For this review, take the finished solid that the model builds, in its own axes (mm). A direction names the side the tool comes from. Round coordinates to 2 decimals unless told otherwise and drop trailing zeros. Put each result on its own line as item: value.
from build123d import *

# Parameters (mm, degrees)
SKETCH_1_W          = 140
SKETCH_1_H          = 20.2
SKETCH_1_R          = 3
SKETCH_1_R_2        = 2.5
EXTRUDE_1_DEPTH     = 5
CUT_EXTRUDE_1_DEPTH = 41


with BuildPart() as part:
    # 스케치1 → 돌출1 (new body)
    with BuildSketch(Plane.XY):
        with Locations((12.953994506, 0)):
            Rectangle(SKETCH_1_W, SKETCH_1_H)
        with Locations((-47.044353904, 0)):
            Circle(SKETCH_1_R, mode=Mode.SUBTRACT)
        with Locations((12.955646096, 0)):
            Circle(SKETCH_1_R, mode=Mode.SUBTRACT)
        with Locations((42.953994506, 0)):
            Circle(SKETCH_1_R_2, mode=Mode.SUBTRACT)
        with Locations((72.953994506, 0)):
            Circle(SKETCH_1_R, mode=Mode.SUBTRACT)
        with BuildLine():
            Line((-16.044353904, 5), (-18.044353904, 5))
            ThreePointArc((-18.044353904, 5), (-23.044353904, 0), (-18.044353904, -5))
            Line((-18.044353904, -5), (-16.044353904, -5))
            ThreePointArc((-16.044353904, -5), (-11.044353904, 0), (-16.044353904, 5))
        make_face(mode=Mode.SUBTRACT)
        with BuildLine():
            Line((-16.044353904, 7.5), (-18.044353904, 7.5))
            ThreePointArc((-18.044353904, 7.5), (-19.044353904, 8.5), (-18.044353904, 9.5))
            Line((-18.044353904, 9.5), (-16.044353904, 9.5))
            ThreePointArc((-16.044353904, 9.5), (-15.044353904, 8.5), (-16.044353904, 7.5))
        make_face(mode=Mode.SUBTRACT)
        with BuildLine():
            Line((-10.683137972, -5.25), (-8.683137972, -5.25))
            ThreePointArc((-8.683137972, -5.25), (-7.683137972, -4.25), (-8.683137972, -3.25))
            Line((-8.683137972, -3.25), (-10.683137972, -3.25))
            ThreePointArc((-10.683137972, -3.25), (-11.683137972, -4.25), (-10.683137972, -5.25))
        make_face(mode=Mode.SUBTRACT)
        with BuildLine():
            Line((-9.620718033, -1), (-7.467989775, -1))
            ThreePointArc((-7.467989775, -1), (-6.543625234, 0.036752017), (-7.544353904, 1))
            Line((-7.544353904, 1), (-9.544353904, 1))
            ThreePointArc((-9.544353904, 1), (-10.545082573, 0.036752017), (-9.620718033, -1))
        make_face(mode=Mode.SUBTRACT)
        with BuildLine():
            Line((-20.294353904, 8.361215932), (-22.294353904, 8.361215932))
            ThreePointArc((-22.294353904, 8.361215932), (-23.294353904, 7.361215932), (-22.294353904, 6.361215932))
            Line((-22.294353904, 6.361215932), (-20.294353904, 6.361215932))
            ThreePointArc((-20.294353904, 6.361215932), (-19.294353904, 7.361215932), (-20.294353904, 8.361215932))
        make_face(mode=Mode.SUBTRACT)
        with BuildLine():
            Line((-23.405569836, 5.25), (-25.405569836, 5.25))
            ThreePointArc((-25.405569836, 5.25), (-26.405569836, 4.25), (-25.405569836, 3.25))
            Line((-25.405569836, 3.25), (-23.405569836, 3.25))
            ThreePointArc((-23.405569836, 3.25), (-22.405569836, 4.25), (-23.405569836, 5.25))
        make_face(mode=Mode.SUBTRACT)
        with BuildLine():
            Line((-24.544353904, 1), (-26.544353904, 1))
            ThreePointArc((-26.544353904, 1), (-27.545082573, 0.036752017), (-26.620718033, -1))
            Line((-26.620718033, -1), (-24.467989775, -1))
            ThreePointArc((-24.467989775, -1), (-23.543625234, 0.036752017), (-24.544353904, 1))
        make_face(mode=Mode.SUBTRACT)
        with BuildLine():
            Line((-10.683137972, 3.25), (-8.683137972, 3.25))
            ThreePointArc((-8.683137972, 3.25), (-7.683137972, 4.25), (-8.683137972, 5.25))
            Line((-8.683137972, 5.25), (-10.683137972, 5.25))
            ThreePointArc((-10.683137972, 5.25), (-11.683137972, 4.25), (-10.683137972, 3.25))
        make_face(mode=Mode.SUBTRACT)
        with BuildLine():
            Line((-13.794353904, 6.361215932), (-11.794353904, 6.361215932))
            ThreePointArc((-11.794353904, 6.361215932), (-10.794353904, 7.361215932), (-11.794353904, 8.361215932))
            Line((-11.794353904, 8.361215932), (-13.794353904, 8.361215932))
            ThreePointArc((-13.794353904, 8.361215932), (-14.794353904, 7.361215932), (-13.794353904, 6.361215932))
        make_face(mode=Mode.SUBTRACT)
        with BuildLine():
            Line((-23.405569836, -3.25), (-25.405569836, -3.25))
            ThreePointArc((-25.405569836, -3.25), (-26.405569836, -4.25), (-25.405569836, -5.25))
            Line((-25.405569836, -5.25), (-23.405569836, -5.25))
            ThreePointArc((-23.405569836, -5.25), (-22.405569836, -4.25), (-23.405569836, -3.25))
        make_face(mode=Mode.SUBTRACT)
        with BuildLine():
            Line((-13.794353904, -8.361215932), (-11.794353904, -8.361215932))
            ThreePointArc((-11.794353904, -8.361215932), (-10.794353904, -7.361215932), (-11.794353904, -6.361215932))
            Line((-11.794353904, -6.361215932), (-13.794353904, -6.361215932))
            ThreePointArc((-13.794353904, -6.361215932), (-14.794353904, -7.361215932), (-13.794353904, -8.361215932))
        make_face(mode=Mode.SUBTRACT)
        with BuildLine():
            Line((-20.294353904, -6.361215932), (-22.294353904, -6.361215932))
            ThreePointArc((-22.294353904, -6.361215932), (-23.294353904, -7.361215932), (-22.294353904, -8.361215932))
            Line((-22.294353904, -8.361215932), (-20.294353904, -8.361215932))
            ThreePointArc((-20.294353904, -8.361215932), (-19.294353904, -7.361215932), (-20.294353904, -6.361215932))
        make_face(mode=Mode.SUBTRACT)
        with BuildLine():
            Line((-16.044353904, -9.5), (-18.044353904, -9.5))
            ThreePointArc((-18.044353904, -9.5), (-19.044353904, -8.5), (-18.044353904, -7.5))
            Line((-18.044353904, -7.5), (-16.044353904, -7.5))
            ThreePointArc((-16.044353904, -7.5), (-15.044353904, -8.5), (-16.044353904, -9.5))
        make_face(mode=Mode.SUBTRACT)
    extrude(amount=EXTRUDE_1_DEPTH)

    # 스케치8 → 컷-돌출1 (cut)
    with BuildSketch(Plane.XZ.offset(10.1)):
        with BuildLine():
            ThreePointArc((77.953994506, 2.5), (79.453994506, 1), (80.953994506, 2.5))
            Line((80.953994506, 2.5), (77.953994506, 2.5))
        make_face()
        with BuildLine():
            Line((77.953994506, 2.5), (80.953994506, 2.5))
            ThreePointArc((80.953994506, 2.5), (79.453994506, 4), (77.953994506, 2.5))
        make_face()
        with BuildLine():
            ThreePointArc((61.453994506, 2.5), (62.953994506, 1), (64.453994506, 2.5))
            Line((64.453994506, 2.5), (61.453994506, 2.5))
        make_face()
        with BuildLine():
            Line((61.453994506, 2.5), (64.453994506, 2.5))
            ThreePointArc((64.453994506, 2.5), (62.953994506, 4), (61.453994506, 2.5))
        make_face()
        with BuildLine():
            ThreePointArc((51.453994506, 2.5), (52.953994506, 1), (54.453994506, 2.5))
            Line((54.453994506, 2.5), (51.453994506, 2.5))
        make_face()
        with BuildLine():
            Line((51.453994506, 2.5), (54.453994506, 2.5))
            ThreePointArc((54.453994506, 2.5), (52.953994506, 4), (51.453994506, 2.5))
        make_face()
        with BuildLine():
            ThreePointArc((31.453994506, 2.5), (32.953994506, 1), (34.453994506, 2.5))
            Line((34.453994506, 2.5), (31.453994506, 2.5))
        make_face()
        with BuildLine():
            Line((31.453994506, 2.5), (34.453994506, 2.5))
            ThreePointArc((34.453994506, 2.5), (32.953994506, 4), (31.453994506, 2.5))
        make_face()
        with BuildLine():
            ThreePointArc((21.453994506, 2.5), (22.953994506, 1), (24.453994506, 2.5))
            Line((24.453994506, 2.5), (21.453994506, 2.5))
        make_face()
        with BuildLine():
            Line((21.453994506, 2.5), (24.453994506, 2.5))
            ThreePointArc((24.453994506, 2.5), (22.953994506, 4), (21.453994506, 2.5))
        make_face()
        with BuildLine():
            ThreePointArc((-1.044353904, 2.5), (0.455646096, 1), (1.955646096, 2.5))
            Line((1.955646096, 2.5), (-1.044353904, 2.5))
        make_face()
        with BuildLine():
            Line((-1.044353904, 2.5), (1.955646096, 2.5))
            ThreePointArc((1.955646096, 2.5), (0.455646096, 4), (-1.044353904, 2.5))
        make_face()
        with BuildLine():
            ThreePointArc((-36.044353904, 2.5), (-34.544353904, 1), (-33.044353904, 2.5))
            Line((-33.044353904, 2.5), (-36.044353904, 2.5))
        make_face()
        with BuildLine():
            Line((-36.044353904, 2.5), (-33.044353904, 2.5))
            ThreePointArc((-33.044353904, 2.5), (-34.544353904, 4), (-36.044353904, 2.5))
        make_face()
        with BuildLine():
            ThreePointArc((-56.044353904, 2.5), (-54.544353904, 1), (-53.044353904, 2.5))
            Line((-53.044353904, 2.5), (-56.044353904, 2.5))
        make_face()
        with BuildLine():
            Line((-56.044353904, 2.5), (-53.044353904, 2.5))
            ThreePointArc((-53.044353904, 2.5), (-54.544353904, 4), (-56.044353904, 2.5))
        make_face()
    extrude(amount=-CUT_EXTRUDE_1_DEPTH, mode=Mode.SUBTRACT)


solid = part.part
(1) Insertion check: pin 1 Ø2.5 at (x, z) = (22.95, 2.5) entering from +Y. The pin has a flat end and moves straight along its axis. Give the tip position at first contact, or say it passes through.
A:
pin 1: passes through
(2) For faces 1 (the face through (12, -10.1, 2)), 2 (the face through (-23.043, 0.11, 2.465)), list the 3-axis set-ups (+Z, -Z, +X, -X, +Y, -Y) from which the entire face can be reached by the end or side of a thin tool; tool diameter is ignored.
A:
face 1: +Z, -Z, +X, -X, -Y
face 2: +Z, -Z
(3) Draft analysis for pull direction Z (two halves, no side actions). For faces 3 (the face through (-9, -1, 2)), 4 (the face through (61.76, -0.14, 1.59)), 5 (the face through (77.955, -0.141, 2.566)), 6 (the face through (12, 5, 0)), state which applies: released by +Z, released by -Z, zero draft, split by the parting line, or undercut.
A:
face 3: zero draft
face 4: undercut
face 5: undercut
face 6: released by -Z
(4) Add section A-A on z = 2.5. State how many separate pieces and enclosed holes the cut face has, then the cut area to 3 significant figures.
A:
separate pieces: 9
enclosed holes: 17
area: 2,050 mm2
(5) To check wall thickness, follow L1, parallel to Y at x = -8.5, z = 1.9; L2, parallel to Z at x = 33, y = -1; L3, parallel to Y at x = -11, z = 1.75. State the ranges of each line that lie inside material, in increasing order.
A:
L1: y = -10.1 to -5.23, -3.27 to -1, 1 to 3.27, 5.23 to 10.1
L2: z = 0 to 1, 4 to 5
L3: y = -10.1 to -7.97, -6.75 to -5.2, -3.3 to 3.3, 5.2 to 6.75, 7.97 to 10.1
